from build123d import *

# Parameters (mm, degrees)
SKETCH001_W     = 31.2
SKETCH001_H     = 78.4
PAD001_DEPTH    = 4
SKETCH002_W     = 31.2
SKETCH002_H     = 78.4
PAD002_DEPTH    = 0.8
SKETCH006_W     = 4
SKETCH006_H     = 2
POCKET001_DEPTH = 5
SKETCH009_W     = 1.4
SKETCH009_H     = 7.45
PAD006_DEPTH    = 2.2
FILLET001_R     = 4


with BuildPart() as part:
    # Sketch001 → Pad001 (new body)
    with BuildSketch(Plane.XY):
        with Locations((15.6, -39.2)):
            Rectangle(SKETCH001_W, SKETCH001_H)
        Polygon((3, -2), (28.2, -2), (28.2, -76.9), (3, -76.9), (3, -70.886093), (1, -70.886093), (1, -57.206394), (3, -57.206394), align=None, mode=Mode.SUBTRACT)
    extrude(amount=PAD001_DEPTH)

    # Sketch002 (on Face14 of Pad001) → Pad002 (join)
    with BuildSketch(Plane.XY.offset(4)):
        with Locations((15.6, -39.2)):
            Rectangle(SKETCH002_W, SKETCH002_H)
    extrude(amount=PAD002_DEPTH)

    # Sketch006 (on Face1 of Pad002) → Pocket001 (cut)
    with BuildSketch(Plane(origin=(0, 0, 0), x_dir=(-1, 0, 0), z_dir=(0, 1, 0))):
        with Locations((-15.6, 1)):
            Rectangle(SKETCH006_W, SKETCH006_H)
    extrude(amount=-POCKET001_DEPTH, mode=Mode.SUBTRACT)

    # Sketch009 (on Face4 of Pad002) → Pad006 (join)
    with BuildSketch(Plane(origin=(0, 0, 0), x_dir=(1, 0, 0), z_dir=(0, 0, -1))):
        with Locations((0.7, 57.125)):
            Rectangle(SKETCH009_W, SKETCH009_H)
        with Locations((0.7, 21.275)):
            Rectangle(SKETCH009_W, SKETCH009_H)
        with Locations((30.5, 21.275)):
            Rectangle(SKETCH009_W, SKETCH009_H)
        with Locations((30.5, 57.125)):
            Rectangle(SKETCH009_W, SKETCH009_H)
    extrude(amount=PAD006_DEPTH)

    # Fillet001
    fillet001_edges = [part.edges().sort_by_distance(p)[0] for p in [
        (0, -78.4, 2),
        (0, 0, 2),
        (31.2, -78.4, 2),
        (31.2, 0, 2),
    ]]
    fillet(fillet001_edges, radius=FILLET001_R)


with BuildPart() as part_1:
    # Body001 placement: moved
    add(part.part.moved(Location((0, 0, 6))))


solid = part_1.part
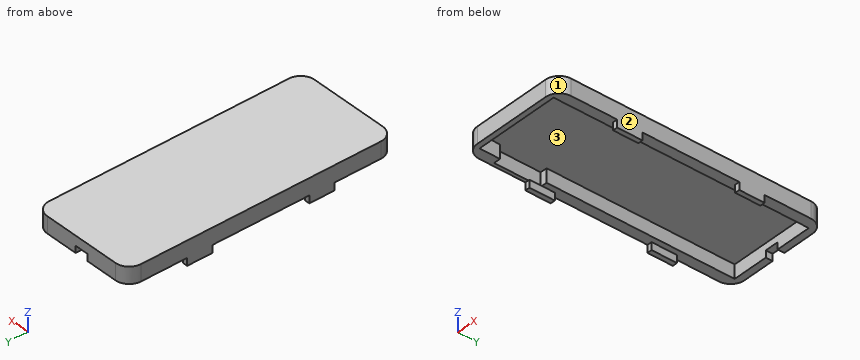
Design review of the part built by this model. Coordinates are the model's own, in mm. Face numbers are marked on the shaded views. Round coordinates to 2 decimals unless told otherwise and drop trailing zeros. Loops run counter-clockwise (first coordinate to the right, second up) from the corner with the lowest first, then second, coordinate; pieces in that order, holes last. Notation, with made-up numbers: (68, 28.5) -> (94, 28.5) arc R16 cw to (94, 57.5) -> close; hole circle Ø3 at (16.25, 51). An arc over 180 degrees is marked (long way). Use one line per item in the form item = value. Start each with the question number.
Q1. We need section B-B on z = 4.5. Give the boundary of the cut face in (x, y).
Q2. We need section D-D on z = 8.75. Give the boundary of the cut face in (x, y), then the cut area to 3 significant figures.
Q3. Draft analysis for pull direction Y (two halves, no side actions). For the marked faces 1, 2 and 3, state which applies: +Y half, -Y half, draft (parallel to the pull), parting line (faces both ways), or undercut.
Q4. Wall thickness on line 1 along X through (y, z) = (-56, 5.75); line 2 along X through (y, z) = (-40.5, 8.25); line 3 along Y through (x, z) = (8, 7): over which ranges is each line inside the solid? List them lowest first. Write a range as [from, to].
Q5. We need section C-C on x = 16.5. Give the boundary of the cut face in (y, z).
Q6. For pin 1 Ø1.5 at (x, z) = (1, 5) entering from -Y; pin 2 Ø1.6 at (x, y) = (15.5, -1) entering from -Z; pin 3 Ø2.5 at (y, z) = (-21, 5) entering from -X; pin 4 Ø15.5 at (x, y) = (11.5, -21.5) entering from -Z, all flat-tipped, find the tip position at first contact; note any pin that passes through.
Q7. We need section A-A on y = -63.5. Give the boundary of the cut face in (x, z).
Calculated:
q1.outline = (0, -60.85) -> (1.4, -60.85) -> (1.4, -53.4) -> (0, -53.4) -> close; (0, -25) -> (1.4, -25) -> (1.4, -17.55) -> (0, -17.55) -> close; (29.8, -60.85) -> (31.2, -60.85) -> (31.2, -53.4) -> (29.8, -53.4) -> close; (29.8, -25) -> (31.2, -25) -> (31.2, -17.55) -> (29.8, -17.55) -> close
q2.outline = (0, -74.4) arc R4 ccw to (4, -78.4) -> (27.2, -78.4) arc R4 ccw to (31.2, -74.4) -> (31.2, -4) arc R4 ccw to (27.2, 0) -> (4, 0) arc R4 ccw to (0, -4) -> close; hole (1, -70.89) -> (3, -70.89) -> (3, -76.9) -> (28.2, -76.9) -> (28.2, -2) -> (3, -2) -> (3, -57.21) -> (1, -57.21) -> close
q2.area = 518 mm²
q3.face_1 = -Y half
q3.face_2 = draft
q3.face_3 = undercut
q4.line_1 = [0, 1.4], [29.8, 31.2]
q4.line_2 = [0, 3], [28.2, 31.2]
q4.line_3 = [-78.4, -76.9], [-2, 0]
q5.outline = (-78.4, 6) -> (-76.9, 6) -> (-76.9, 10) -> (-2, 10) -> (-2, 8) -> (0, 8) -> (0, 10.8) -> (-78.4, 10.8) -> close
q6.pin_1 = -60.85
q6.pin_2 = 8
q6.pin_3 = 0
q6.pin_4 = 10
q7.outline = (0, 6) -> (1, 6) -> (1, 10) -> (28.2, 10) -> (28.2, 6) -> (31.2, 6) -> (31.2, 10.8) -> (0, 10.8) -> close
